```python
from build123d import *

# Parameters (mm, degrees)
CUT_EXTRUDE1_REACH = 46.685
SKETCH2_R          = 7.366


with BuildPart() as part:
    # Sketch1 → Revolve1 (revolve)
    with BuildSketch(Plane(origin=(0, 0, 0), x_dir=(0, 0, -1), z_dir=(1, 0, 0)), mode=Mode.PRIVATE) as revolve1_sk:
        Polygon((0, 0), (-16.51, 0), (-16.51, 38.1), (-8.9281, 38.1), (-8.9281, 20.32), (-10.795, 20.32), (-10.795, 2.54), (-8.9281, 2.54), (0, 2.54), align=None)
    revolve(revolve1_sk.sketch.rotate(Axis((0, 0, 0), (0, 1, 0)), 180), axis=Axis((0, 0, 0), (0, 1, 0)))

    # Sketch2 → Cut-Extrude1 (cut, up to next)
    with BuildSketch(Plane.XZ, mode=Mode.PRIVATE) as cut_extrude1_sk1:
        with Locations(Location((0, 0, 0), (0, 0, 270))):
            Circle(SKETCH2_R)
    cut_extrude1_tool1 = extrude(cut_extrude1_sk1.sketch, amount=-CUT_EXTRUDE1_REACH, mode=Mode.PRIVATE) & part.part
    add(cut_extrude1_tool1.solids().sort_by_distance((0, 0, 0))[0], mode=Mode.SUBTRACT)


solid = part.part
```
Read the model definition and answer for the solid it produces. Units are mm, in the model's axes. A direction names the side the tool comes from. Give positions to 0.01 mm unless a question says otherwise; leave off trailing zeros. Order: outer loops, then holes, each group sorted by start corner. A loop starts at its lowest first (then second) coordinate and runs counter-clockwise, first axis right, second up.
(1) Find section B-B (x = 0). Give the vertices of the cut face in (y, z) (3 decimals).
(2) Straight lines are drawn through the part: L1, parallel to Y at x = -1.5, z = 10; L2, parallel to Z at x = -3, y = 11.5; L3, parallel to X at y = 10, z = 0 (3 decimals). For each, find the intervals that lie inside material, in ascending order.
(3) Find section A-A (z = 0). Give the vertices of the cut face in (x, y) (3 decimals), plus the area to 3 significant figures.
(4) Given pin 1 (6.5 mm diameter, centred on x = 0.5, z = 5, fed in from +Y); pin 2 (10 mm diameter, centred on x = -10, y = 24.5, fed in from +Z); pin 3 (4 mm diameter, centred on x = -10, y = 25, fed in from -Z), each flat-ended and moving along its own axis, determine where each tip first touches the part or whether it passes through.
(5) Find section D-D (z = -8). Give the vertices of the cut face in (x, y).
(6) For faces 1 (the flat face through (7, 38.1, -7)), 2 (the cylindrical face through (-2.682, 29.086, -8.516)), 3 (the flat face through (7, 2.54, -3)), determine the directions among +Z, -Z, +X, -X, +Y, -Y from which every point of the face is accessible in a straight line to the end or side of a thin tool.
(7) Find section C-C (y = 16). Give the vertices of the cut face in (x, z) (3 decimals), plus the area to 3 significant figures.
(8) For a pull along Z with two mould halves and no side action, classify faces 4 (the cylindrical face through (-6.535, 1.252, -3.399)), 5 (the flat face through (7, 0, 3)), 6 (the cylindrical face through (-4.959, 19.317, -15.748)), 7 (the flat face through (-9, 20.32, 2)) as released by +Z, released by -Z, zero draft, split by the parting line, or undercut.
Result sheet:
1. outline: (0, -16.51) - (38.1, -16.51) - (38.1, -8.928) - (20.32, -8.928) - (20.32, -10.795) - (2.54, -10.795) - (2.54, -7.366) - (0, -7.366) - close; (0, 7.366) - (2.54, 7.366) - (2.54, 10.795) - (20.32, 10.795) - (20.32, 8.928) - (38.1, 8.928) - (38.1, 16.51) - (0, 16.51) - close
2. L1: y = 0 to 2.54, 20.32 to 38.1
2. L2: z = -16.24 to -10.37, 10.37 to 16.24
2. L3: x = -16.51 to -10.795, 10.795 to 16.51
3. outline: (-16.51, 0) - (-7.366, 0) - (-7.366, 2.54) - (-10.795, 2.54) - (-10.795, 20.32) - (-8.928, 20.32) - (-8.928, 38.1) - (-16.51, 38.1) - close; (7.366, 0) - (16.51, 0) - (16.51, 38.1) - (8.928, 38.1) - (8.928, 20.32) - (10.795, 20.32) - (10.795, 2.54) - (7.366, 2.54) - close
3. area: 519 mm2
4. pin 1: stops at y = 2.54
4. pin 2: stops at z = 15.73
4. pin 3: stops at z = -14.44
5. outline: (-14.44, 0) - (14.44, 0) - (14.44, 38.1) - (3.96, 38.1) - (3.96, 20.32) - (7.25, 20.32) - (7.25, 2.54) - (-7.25, 2.54) - (-7.25, 20.32) - (-3.96, 20.32) - (-3.96, 38.1) - (-14.44, 38.1) - close
6. face 1: +Z, -Z, +X, -X, +Y
6. face 2: +Y
6. face 3: none
7. outline: circle Ø33.02 at (0, 0); hole circle Ø21.59 at (0, 0)
7. area: 490 mm2
8. face 4: undercut
8. face 5: zero draft
8. face 6: split by the parting line
8. face 7: undercut
